Build history of the part. All positions in model axes, mm. Coordinates: 2 decimals unless noted, no trailing zeros. Order: outer loops, then holes, each group sorted by start corner. A loop starts at its lowest first (then second) coordinate and runs counter-clockwise, first axis right, second up. Notation, with made-up numbers: (79, 57.5) - (138, 57.5) arc R12 ccw to (138, 72.5) - close; hole circle Ø7 at (53.25, 18). An arc over 180 degrees is marked (long way). Return JSON: item names as keys, results as strings.
from build123d import *

# Parameters (mm, degrees)
SKETCH1_R           = 2.0955
BOSS_EXTRUDE1_DEPTH = 1.27
FILLET1_R           = 6.35
FILLET2_R           = 101.6


with BuildPart() as part:
    # Sketch1 → Boss-Extrude1 (new, symmetric)
    with BuildSketch(Plane(origin=(0, 0, 0), x_dir=(0, 0, -1), z_dir=(1, 0, 0))):
        Polygon((-138.948360469, -3.051094372), (140.451639531, -3.051094372), (140.451639531, 151.896865158), (174.673969175, 195.068905628), (-108.718972293, 195.068905628), (-138.948360469, 151.896865158), align=None)
        with Locations((-113.548360469, 4.568905628)):
            Circle(SKETCH1_R, mode=Mode.SUBTRACT)
        with Locations((-88.148360469, 4.568905628)):
            Circle(SKETCH1_R, mode=Mode.SUBTRACT)
        with Locations((-62.748360469, 4.568905628)):
            Circle(SKETCH1_R, mode=Mode.SUBTRACT)
        with Locations((-37.348360469, 4.568905628)):
            Circle(SKETCH1_R, mode=Mode.SUBTRACT)
        with Locations((-11.948360469, 4.568905628)):
            Circle(SKETCH1_R, mode=Mode.SUBTRACT)
        with Locations((13.451639531, 4.568905628)):
            Circle(SKETCH1_R, mode=Mode.SUBTRACT)
        with Locations((38.851639531, 4.568905628)):
            Circle(SKETCH1_R, mode=Mode.SUBTRACT)
        with Locations((64.251639531, 4.568905628)):
            Circle(SKETCH1_R, mode=Mode.SUBTRACT)
        with Locations((89.651639531, 4.568905628)):
            Circle(SKETCH1_R, mode=Mode.SUBTRACT)
        with Locations((115.051639531, 4.568905628)):
            Circle(SKETCH1_R, mode=Mode.SUBTRACT)
        with Locations((-96.018972293, 187.448905628)):
            Circle(SKETCH1_R, mode=Mode.SUBTRACT)
        with Locations((-70.618972293, 187.448905628)):
            Circle(SKETCH1_R, mode=Mode.SUBTRACT)
        with Locations((-45.218972293, 187.448905628)):
            Circle(SKETCH1_R, mode=Mode.SUBTRACT)
        with Locations((-19.818972293, 187.448905628)):
            Circle(SKETCH1_R, mode=Mode.SUBTRACT)
        with Locations((5.581027707, 187.448905628)):
            Circle(SKETCH1_R, mode=Mode.SUBTRACT)
        with Locations((30.981027707, 187.448905628)):
            Circle(SKETCH1_R, mode=Mode.SUBTRACT)
        with Locations((56.381027707, 187.448905628)):
            Circle(SKETCH1_R, mode=Mode.SUBTRACT)
        with Locations((81.781027707, 187.448905628)):
            Circle(SKETCH1_R, mode=Mode.SUBTRACT)
        with Locations((107.181027707, 187.448905628)):
            Circle(SKETCH1_R, mode=Mode.SUBTRACT)
        with Locations((132.581027707, 187.448905628)):
            Circle(SKETCH1_R, mode=Mode.SUBTRACT)
        with Locations((157.981027707, 187.448905628)):
            Circle(SKETCH1_R, mode=Mode.SUBTRACT)
    extrude(amount=BOSS_EXTRUDE1_DEPTH, both=True)

    # Fillet1
    fillet1_edges = [part.edges().sort_by_distance(p)[0] for p in [
        (0, -3.051094372, -140.451639531),
        (0, -3.051094372, 138.948360469),
        (0, 195.068905628, 108.718972293),
        (0, 195.068905628, -174.673969175),
    ]]
    fillet(fillet1_edges, radius=FILLET1_R)

    # Fillet2
    fillet2_edges = [part.edges().sort_by_distance(p)[0] for p in [
        (0, 151.896865158, -140.451639531),
        (0, 151.896865158, 138.948360469),
    ]]
    fillet(fillet2_edges, radius=FILLET2_R)


solid = part.part
1. Cut at C-C on y = 123.5. Give the cut face in (x, z), plus the area to 3 significant figures.
Check values:
{"outline": "(-1.27, -140.69) - (1.27, -140.69) - (1.27, 138.88) - (-1.27, 138.88) - close", "area": "710 mm²"}
2. Drop a flat-ended pin along its axis: pin 1 (3.5 mm diameter, centred on y = 4.57, z = -38.85, fed in from -X). Give the stop position or say it passes through.
Check values:
{"pin 1": "through"}
3. Cut at B-B on y = 29. Give the cut face in (x, z).
Check values:
{"outline": "(-1.27, -140.45) - (1.27, -140.45) - (1.27, 138.95) - (-1.27, 138.95) - close"}
4. Cut at A-A on x = -0.5. State how many separate pieces and enclosed holes the cut face has, plus the area to 3 significant figures.
Check values:
{"separate pieces": "1", "enclosed holes": "21", "area": "55,100 mm²"}
5. Probe L1, parallel to Y at x = 0.85, z = -54.5; L2, parallel to Z at x = 0.85, y = 18; L3, parallel to Y at x = 0.5, z = -7.5. List the from-to ranges inside material, lowest first.
Check values:
{"L1": "-3.05 to 186.53, 188.37 to 195.07", "L2": "-140.45 to 138.95", "L3": "-3.05 to 186.61, 188.29 to 195.07"}
